Input: part model. Units: mm. Frame: model coordinates. Face numbers are marked on the shaded views. Round coordinates to 2 decimals unless told otherwise and drop trailing zeros. Loops run counter-clockwise (first coordinate to the right, second up) from the corner with the lowest first, then second, coordinate; pieces in that order, holes last. Notation, with made-up numbers: M -30.75,-3.5 L 2.25,-3.5 A18 cw 2.25,13.5 Z; hole C 9.5,9 d2. An arc over 180 degrees is marked long. Put each result on its own line as item: value. Start each with the question number.
1) Draft query along X for the marked faces 1 and 2. Return one class per face: +X half, -X half, draft (parallel to the pull), parting line (faces both ways), or undercut.
2) Section A-A on y = -2. Output: boundary loops of the cut face in (x, z), plus the area to 3 significant figures.
3) Section B-B on x = -0.5. Output: boundary loops of the cut face in (y, z).
4) Section C-C on z = 10.5. Output: boundary loops of the cut face in (x, y).
5) Pin query (flat end, axial travel): pin 1 (0.9 mm diameter, centred on y = -1.5, z = 7.5, fed in from -X); pin 2 (0.6 mm diameter, centred on x = -22, y = -1.5, fed in from +Z); pin 3 (0.9 mm diameter, centred on x = -3, y = -2, fed in from +Z). Return the tip coordinate at first contact, or that it passes through.
6) Line query: probe 1 along Z at (x, y) = (-13.5, -2.15); probe 2 along X at (y, z) = (-1.75, 7.75); probe 3 along X at (y, z) = (-1.2, 8.25). Output: solid intervals per line, ascending.
from build123d import *

# Parameters (mm, degrees)
F1_DEPTH = 3
F2_DEPTH = 3


with BuildPart() as f1:
    # F0 (on Front) → F1 (new body)
    with BuildSketch(Plane.XZ):
        with BuildLine():
            Line((-24.701704, 2.93977), (-24.701704, 0))
            Line((-24.701704, 0), (-21.494682, 0))
            Line((-21.494682, 0), (-19.878102, 0))
            ThreePointArc((-19.878102, 0), (-14.698851, -3.900059), (-9.519599, 0))
            Line((-9.519599, 0), (0, -3.397916))
            Line((0, -3.397916), (0, 0))
            Line((0, 0), (19.738455, -3.245201))
            Line((19.738455, -3.245201), (19.738455, 14.08799))
            Line((19.738455, 14.08799), (0, 9.888318))
            Line((0, 9.888318), (-1.695249, 9.888318))
            Line((-1.695249, 9.888318), (-1.695249, 3.388318))
            Line((-1.695249, 3.388318), (-4.595249, 3.388318))
            Line((-4.595249, 3.388318), (-4.595249, 9.888318))
            Line((-4.595249, 9.888318), (-6.604938, 9.888318))
            Line((-6.604938, 9.888318), (-18.516734, 3.092485))
            Line((-18.516734, 3.092485), (-18.207028, 2.176193))
            Line((-18.207028, 2.176193), (-21.128689, 1.495096))
            Line((-21.128689, 1.495096), (-21.57104, 2.176193))
            Line((-21.57104, 2.176193), (-23.709055, 2.176193))
            Line((-23.709055, 2.176193), (-24.701704, 2.93977))
        make_face()
    extrude(amount=F1_DEPTH)

    # F0 (on Front) → F2 (join)
    with BuildSketch(Plane.XZ):
        with BuildLine():
            Line((-24.701704, 2.93977), (-24.701704, 0))
            Line((-24.701704, 0), (-21.494682, 0))
            Line((-21.494682, 0), (-19.878102, 0))
            ThreePointArc((-19.878102, 0), (-14.698851, -3.900059), (-9.519599, 0))
            Line((-9.519599, 0), (0, -3.397916))
            Line((0, -3.397916), (0, 0))
            Line((0, 0), (19.738455, -3.245201))
            Line((19.738455, -3.245201), (19.738455, 14.08799))
            Line((19.738455, 14.08799), (0, 9.888318))
            Line((0, 9.888318), (-1.695249, 9.888318))
            Line((-1.695249, 9.888318), (-1.695249, 3.388318))
            Line((-1.695249, 3.388318), (-4.595249, 3.388318))
            Line((-4.595249, 3.388318), (-4.595249, 9.888318))
            Line((-4.595249, 9.888318), (-6.604938, 9.888318))
            Line((-6.604938, 9.888318), (-18.516734, 3.092485))
            Line((-18.516734, 3.092485), (-18.207028, 2.176193))
            Line((-18.207028, 2.176193), (-21.128689, 1.495096))
            Line((-21.128689, 1.495096), (-21.57104, 2.176193))
            Line((-21.57104, 2.176193), (-23.709055, 2.176193))
            Line((-23.709055, 2.176193), (-24.701704, 2.93977))
        make_face()
    extrude(amount=F2_DEPTH)


solid = f1.part
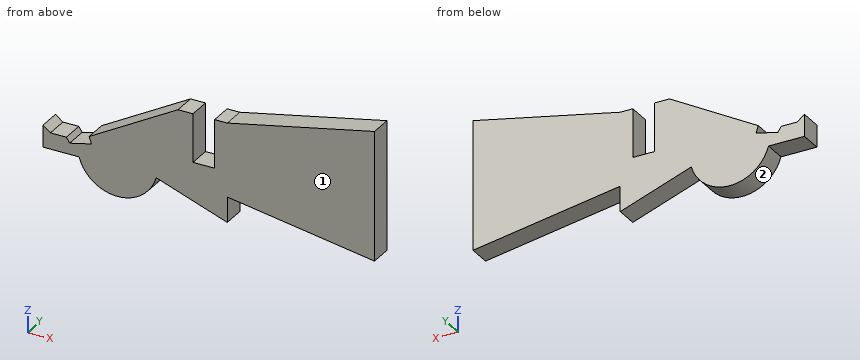
Geometry results:
1. face 1: draft
1. face 2: undercut
2. outline: M -24.7,0 L -19.88,0 A5.39 ccw -9.52,0 L 0,-3.4 L 0,0 L 19.74,-3.25 L 19.74,14.09 L 0,9.89 L -1.7,9.89 L -1.7,3.39 L -4.6,3.39 L -4.6,9.89 L -6.6,9.89 L -18.52,3.09 L -18.21,2.18 L -21.13,1.5 L -21.57,2.18 L -23.71,2.18 L -24.7,2.94 Z
2. area: 451 mm²
3. outline: M -3,-3.22 L 0,-3.22 L 0,9.89 L -3,9.89 Z
4. outline: M 2.87,-3 L 19.74,-3 L 19.74,0 L 2.87,0 Z
5. pin 1: stops at x = -11.58
5. pin 2: stops at z = 2.18
5. pin 3: stops at z = 3.39
6. probe 1: z = -3.77 to 5.95
6. probe 2: x = -10.35 to -4.6, -1.7 to 19.74
6. probe 3: x = -9.48 to -4.6, -1.7 to 19.74
